Check sheet for the modelled part. Datum: model origin and axes. Units: mm. Face numbers are marked on the shaded views. A direction names the side the tool comes from. Round coordinates to 2 decimals unless told otherwise and drop trailing zeros. Loops run counter-clockwise (first coordinate to the right, second up) from the corner with the lowest first, then second, coordinate; pieces in that order, holes last. Notation, with made-up numbers: (-18.5, 58) - (0.5, 58) arc R38 ccw to (0.5, 96) - close; hole circle Ø7 at (-15.75, -31.5). An arc over 180 degrees is marked (long way). Put each result on its own line as item: value.
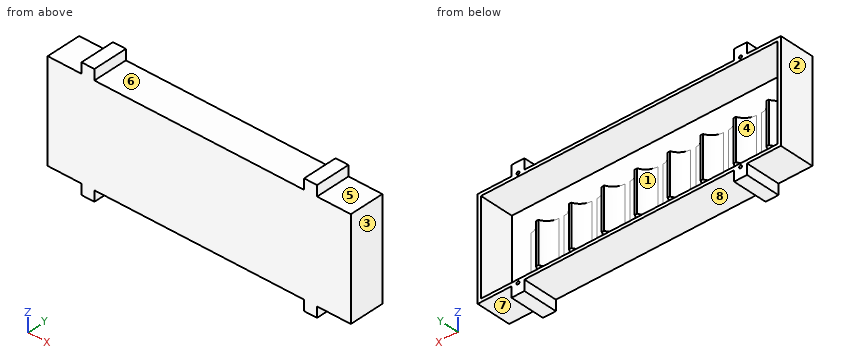
```python
from build123d import *

# Parameters (mm, degrees)
SKETCH1_W                 = 239.08
SKETCH1_H                 = 78.74
BOSS_EXTRUDE1_DEPTH       = 0.508
SKETCH1_3_W               = 239.08
SKETCH1_3_H               = 8.255
SKETCH1_3_H_2             = 78.74
SKETCH1_3_W_2             = 234
SKETCH1_3_H_3             = 73.66
BOSS_EXTRUDE2_DEPTH       = 27
BOSS_EXTRUDE3_START       = 21.59
BOSS_EXTRUDE3_DEPTH       = 32.5
SKETCH1_4_W               = 239.08
SKETCH1_4_H               = 8.255
BOSS_EXTRUDE4_DEPTH       = 0.508
F_4_40_TAPPED_HOLE2_D     = 2.2606
F_4_40_TAPPED_HOLE2_DEPTH = 7.62
F_4_40_TAPPED_HOLE2_TIP   = 0.679152758
SKETCH13_W                = 165.42
SKETCH13_H                = 8.255
SKETCH13_W_2              = 26.67
CUT_EXTRUDE1_DEPTH        = 28.508


with BuildPart() as part:
    # Sketch1 → Boss-Extrude1 (new body)
    with BuildSketch(Plane(origin=(0, 0, 0), x_dir=(1, 0, 0), z_dir=(0, 1, 0))):
        with Locations((119.54, -39.37)):
            Rectangle(SKETCH1_W, SKETCH1_H)
    extrude(amount=-BOSS_EXTRUDE1_DEPTH)

    # Sketch1<3> → Boss-Extrude2 (add)
    with BuildSketch(Plane(origin=(0, 0, 0), x_dir=(1, 0, 0), z_dir=(0, 1, 0))):
        with Locations((119.54, 4.1275)):
            Rectangle(SKETCH1_3_W, SKETCH1_3_H)
        with Locations((119.54, -82.8675)):
            Rectangle(SKETCH1_3_W, SKETCH1_3_H)
        with Locations((119.54, -39.37)):
            Rectangle(SKETCH1_3_W, SKETCH1_3_H_2)
        with Locations((119.54, -39.37)):
            Rectangle(SKETCH1_3_W_2, SKETCH1_3_H_3, mode=Mode.SUBTRACT)
    extrude(amount=BOSS_EXTRUDE2_DEPTH)

    # Sketch5 → Boss-Extrude3 (add)
    with BuildSketch(Plane.XY.offset(2.54).offset(BOSS_EXTRUDE3_START)):
        with BuildLine():
            Line((29.54, 7), (27.54, 7))
            ThreePointArc((27.54, 7), (23.600043647, 1.985651932), (17.54, 0))
            Line((17.54, 0), (39.54, 0))
            ThreePointArc((39.54, 0), (33.479956353, 1.985651932), (29.54, 7))
        make_face()
        with BuildLine():
            Line((55.4988, 7), (53.4988, 7))
            ThreePointArc((53.4988, 7), (49.558843647, 1.985651932), (43.4988, 0))
            Line((43.4988, 0), (65.4988, 0))
            ThreePointArc((65.4988, 0), (59.438756353, 1.985651932), (55.4988, 7))
        make_face()
        with BuildLine():
            Line((81.4576, 7), (79.4576, 7))
            ThreePointArc((79.4576, 7), (75.517643647, 1.985651932), (69.4576, 0))
            Line((69.4576, 0), (91.4576, 0))
            ThreePointArc((91.4576, 0), (85.397556353, 1.985651932), (81.4576, 7))
        make_face()
        with BuildLine():
            Line((107.4164, 7), (105.4164, 7))
            ThreePointArc((105.4164, 7), (101.476443647, 1.985651932), (95.4164, 0))
            Line((95.4164, 0), (117.4164, 0))
            ThreePointArc((117.4164, 0), (111.356356353, 1.985651932), (107.4164, 7))
        make_face()
        with BuildLine():
            Line((133.3752, 7), (131.3752, 7))
            ThreePointArc((131.3752, 7), (127.435243647, 1.985651932), (121.3752, 0))
            Line((121.3752, 0), (143.3752, 0))
            ThreePointArc((143.3752, 0), (137.315156353, 1.985651932), (133.3752, 7))
        make_face()
        with BuildLine():
            Line((159.334, 7), (157.334, 7))
            ThreePointArc((157.334, 7), (153.394043647, 1.985651932), (147.334, 0))
            Line((147.334, 0), (169.334, 0))
            ThreePointArc((169.334, 0), (163.273956353, 1.985651932), (159.334, 7))
        make_face()
        with BuildLine():
            Line((185.2928, 7), (183.2928, 7))
            ThreePointArc((183.2928, 7), (179.352843647, 1.985651932), (173.2928, 0))
            Line((173.2928, 0), (195.2928, 0))
            ThreePointArc((195.2928, 0), (189.232756353, 1.985651932), (185.2928, 7))
        make_face()
        with BuildLine():
            Line((211.2516, 7), (209.2516, 7))
            ThreePointArc((209.2516, 7), (205.311643647, 1.985651932), (199.2516, 0))
            Line((199.2516, 0), (221.2516, 0))
            ThreePointArc((221.2516, 0), (215.191556353, 1.985651932), (211.2516, 7))
        make_face()
    extrude(amount=BOSS_EXTRUDE3_DEPTH)

    # Sketch1<4> → Boss-Extrude4 (add)
    with BuildSketch(Plane(origin=(0, 0, 0), x_dir=(1, 0, 0), z_dir=(0, 1, 0))):
        with Locations((119.54, 4.1275)):
            Rectangle(SKETCH1_4_W, SKETCH1_4_H)
        with Locations((119.54, -82.8675)):
            Rectangle(SKETCH1_4_W, SKETCH1_4_H)
    extrude(amount=-BOSS_EXTRUDE4_DEPTH)

    # #4-40 Tapped Hole2
    with Locations(Plane(origin=(0, 27, 0), x_dir=(-1, 0, 0), z_dir=(0, 1, 0))):
        with Locations((-31.75, 0), (-207.33, 0), (-31.75, 78.74), (-207.33, 78.74)):
            Hole(F_4_40_TAPPED_HOLE2_D / 2, depth=F_4_40_TAPPED_HOLE2_DEPTH)
            with Locations((0, 0, -(F_4_40_TAPPED_HOLE2_DEPTH + F_4_40_TAPPED_HOLE2_TIP / 2))):  # 118° drill point
                Cone(0, F_4_40_TAPPED_HOLE2_D / 2, F_4_40_TAPPED_HOLE2_TIP, mode=Mode.SUBTRACT)

    # Sketch13 → Cut-Extrude1 (cut, through all)
    with BuildSketch(Plane(origin=(0, 27, 0), x_dir=(1, 0, 0), z_dir=(0, 1, 0))):
        with Locations((119.54, 4.1275)):
            Rectangle(SKETCH13_W, SKETCH13_H)
        with Locations((119.54, -82.8675)):
            Rectangle(SKETCH13_W, SKETCH13_H)
        with Locations((13.335, 4.1275)):
            Rectangle(SKETCH13_W_2, SKETCH13_H)
        with Locations((225.745, 4.1275)):
            Rectangle(SKETCH13_W_2, SKETCH13_H)
        with Locations((225.745, -82.8675)):
            Rectangle(SKETCH13_W_2, SKETCH13_H)
        with Locations((13.335, -82.8675)):
            Rectangle(SKETCH13_W_2, SKETCH13_H)
    extrude(amount=-CUT_EXTRUDE1_DEPTH, mode=Mode.SUBTRACT)


solid = part.part
```
Item 1: Go/stop test with flat-tipped pins: pin 1 (8 mm diameter, centred on x = 117, y = 11.5, fed in from -Z); pin 2 (6.5 mm diameter, centred on y = 18.5, z = 83, fed in from +X); pin 3 (9 mm diameter, centred on y = 8.5, z = 84, fed in from -X). Record where each tip stops, or that it passes through.
Filled sheet:
pin 1: z = 0
pin 2: x = 212.41
pin 3: x = 26.67
Item 2: Section check B-B on x = 152. Enter the section's corners in (y, z).
Filled sheet:
outline: (-0.51, 0) - (27, 0) - (27, 2.54) - (0, 2.54) - (0, 24.13) - (1.16, 24.13) - (1.16, 56.63) - (0, 56.63) - (0, 76.2) - (27, 76.2) - (27, 78.74) - (-0.51, 78.74) - close
Item 3: Section check A-A on y = 23. Enter the section's corners in (x, z) (3 decimals).
Filled sheet:
outline: (0, 0) - (26.67, 0) - (26.67, -8.255) - (36.83, -8.255) - (36.83, 0) - (202.25, 0) - (202.25, -8.255) - (212.41, -8.255) - (212.41, 0) - (239.08, 0) - (239.08, 78.74) - (212.41, 78.74) - (212.41, 86.995) - (202.25, 86.995) - (202.25, 78.74) - (36.83, 78.74) - (36.83, 86.995) - (26.67, 86.995) - (26.67, 78.74) - (0, 78.74) - close; hole (2.54, 2.54) - (236.54, 2.54) - (236.54, 76.2) - (2.54, 76.2) - close; hole circle Ø2.261 at (31.75, 0); hole circle Ø2.261 at (31.75, 78.74); hole circle Ø2.261 at (207.33, 0); hole circle Ø2.261 at (207.33, 78.74)
Item 4: Thickness scan on line 1 (Z direction, x = 31.75, y = 21.25) (3 decimals); line 2 (X direction, y = 22.5, z = 23.5); line 3 (Z direction, x = 157, y = 14.5). Record the ranges inside material, lowest first. Write a range as from..to.
Filled sheet:
line 1: -8.255..-1.13, 1.13..2.54, 76.2..77.61, 79.87..86.995
line 2: 0..2.54, 236.54..239.08
line 3: 0..2.54, 76.2..78.74
Item 5: Release check for a two-part mould opening along X. For the marked faces 1, 2 and 3 record: +X half, -X half, draft (parallel to the pull), parting line (faces both ways), or undercut.
Filled sheet:
face 1: undercut
face 2: -X half
face 3: +X half
Item 6: Section check C-C on z = 73.5. Enter the section's corners in (x, y), then the cut area to 3 significant figures.
Filled sheet:
outline: (0, -0.51) - (239.08, -0.51) - (239.08, 27) - (236.54, 27) - (236.54, 0) - (2.54, 0) - (2.54, 27) - (0, 27) - close
area: 259 mm²
Item 7: Tool access check on the marked faces 4, 5, 6, 7 and 8. Record the directions out of +Z, -Z, +X, -X, +Y, -Y that give a thin tool (end or side, any length) a straight path to the whole face; none if there is none.
Filled sheet:
face 4: +Y
face 5: +Z, +X, +Y, -Y
face 6: +Z, +Y, -Y
face 7: -Z, +X, +Y, -Y
face 8: -Z, +Y, -Y
